Work out the finished part from the listing and answer in its coordinate system (mm). A direction names the side the tool comes from. Round coordinates to 2 decimals unless told otherwise and drop trailing zeros. Loops run counter-clockwise (first coordinate to the right, second up) from the corner with the lowest first, then second, coordinate; pieces in that order, holes last. Notation, with made-up numbers: M -6,60 L 3,60 A28 ccw 3,91 Z; hole C 75.5,46.5 d6. An arc over 180 degrees is marked long. One line per item, written item: value.
```python
from build123d import *

# Parameters (mm, degrees)
F0_W     = 96.52
F0_H     = 76.2
F1_DEPTH = 96.52
F2_T     = -2.54


with BuildPart() as f1:
    # F0 (on Front) → F1 (new body)
    with BuildSketch(Plane.XZ):
        with Locations((6.01927, 26.454038)):
            Rectangle(F0_W, F0_H)
    extrude(amount=F1_DEPTH)

    # F2
    f2_openings = [f1.faces().sort_by_distance(p)[0] for p in [
        (6.01927, -48.26, 64.554038),
    ]]
    offset(amount=F2_T, openings=f2_openings)


solid = f1.part
```
1) Find the intervals of material crossed by probe 1 along X at (y, z) = (-7.5, 36); probe 2 along Y at (x, z) = (38.5, 42.5); probe 3 along Z at (x, y) = (41, -63.5), in increasing order. Write a range as from..to.
Check values:
probe 1: -42.24..-39.7, 51.74..54.28
probe 2: -96.52..-93.98, -2.54..0
probe 3: -11.65..-9.11
2) Find section C-C (y = -59). Give the vertices of the cut face in (x, z), then the cut area to 3 significant figures.
Check values:
outline: M -42.24,-11.65 L 54.28,-11.65 L 54.28,64.55 L 51.74,64.55 L 51.74,-9.11 L -39.7,-9.11 L -39.7,64.55 L -42.24,64.55 Z
area: 619 mm2
3) For faces 1 (the face through (51.739, -48, 27)), 2 (the face through (5, -96.52, 27)), determine the directions among +Z, -Z, +X, -X, +Y, -Y from which every point of the face is accessible in a straight line to the end or side of a thin tool.
Check values:
face 1: +Z
face 2: +Z, -Z, +X, -X, -Y
4) The mould has two halves that part along X. Classify faces 3 (the face through (5, -2.54, 28)), 4 (the face through (5, -48, -9.106)), 5 (the face through (5, -48, -11.646)), 6 (the face through (54.279, -48, 26)): +X half, -X half, draft (parallel to the pull), parting line (faces both ways), or undercut.
Check values:
face 3: undercut
face 4: undercut
face 5: draft
face 6: +X half
5) Find section A-A (z = -3.5). Give the vertices of the cut face in (x, y), then the cut area to 3 significant figures.
Check values:
outline: M -42.24,-96.52 L 54.28,-96.52 L 54.28,0 L -42.24,0 Z; hole M -39.7,-93.98 L 51.74,-93.98 L 51.74,-2.54 L -39.7,-2.54 Z
area: 955 mm2
6) Find section B-B (x = -15). Give the vertices of the cut face in (y, z).
Check values:
outline: M -96.52,-11.65 L 0,-11.65 L 0,64.55 L -2.54,64.55 L -2.54,-9.11 L -93.98,-9.11 L -93.98,64.55 L -96.52,64.55 Z
7) Each of these flat-tipped pins is pushed along its axis until it touches: pin 1 (1 mm diameter, centred on x = -19, y = -23.5, fed in from +Z); pin 2 (2 mm diameter, centred on x = 34.5, z = 31.5, fed in from +Y). Where does it stop, or does it pass through?
Check values:
pin 1: z = -9.11
pin 2: y = 0
